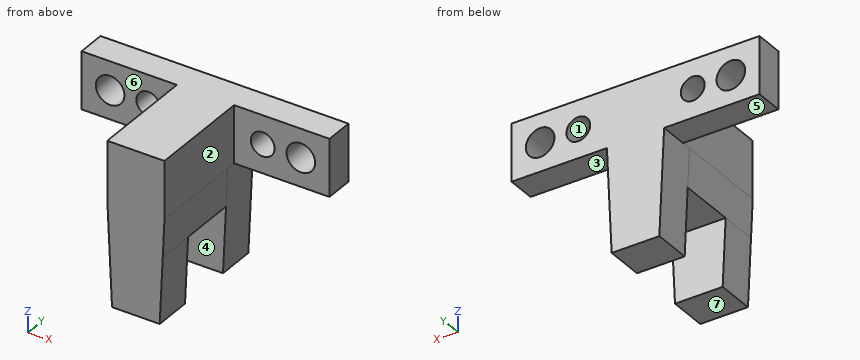
from build123d import *

# Parameters (mm, degrees)
SKETCH_1_W      = 26
SKETCH_1_H      = 6
SKETCH_1_R      = 1.5
SKETCH_1_R_2    = 1.25
EXTRUDE_1_DEPTH = 3
EXTRUDE_2_DEPTH = 4
EXTRUDE_3_DEPTH = 11
EXTRUDE_4_DEPTH = 4


with BuildPart() as part:
    # 草图1 → 凸台-拉伸1 (new body)
    with BuildSketch(Plane(origin=(0, 0, 0), x_dir=(1, 0, 0), z_dir=(0, 1, 0))):
        Rectangle(SKETCH_1_W, SKETCH_1_H)
        with Locations(Location((-10, 0, 0), (0, 0, 270))):
            Circle(SKETCH_1_R, mode=Mode.SUBTRACT)
        with Locations(Location((-6, 0, 0), (0, 0, 270))):
            Circle(SKETCH_1_R_2, mode=Mode.SUBTRACT)
        with Locations(Location((10, 0, 0), (0, 0, 270))):
            Circle(SKETCH_1_R, mode=Mode.SUBTRACT)
        with Locations(Location((6, 0, 0), (0, 0, 270))):
            Circle(SKETCH_1_R_2, mode=Mode.SUBTRACT)
    extrude(amount=EXTRUDE_1_DEPTH)

    # 草图2 → 凸台-拉伸2 (add)
    with BuildSketch(Plane(origin=(0, 3, 0), x_dir=(1, 0, 0), z_dir=(0, 1, 0))):
        Polygon((0, 14), (0, 3), (3, 3), (2.5, 14), align=None)
        Polygon((-3, 3), (0, 3), (0, 14), (-2.5, 14), align=None)
    extrude(amount=-EXTRUDE_2_DEPTH)

    # 草图3 → 凸台-拉伸3 (add)
    with BuildSketch(Plane.XZ):
        Polygon((2.818181818, -7), (3, -3), (0, -3), (0, -7), align=None)
        Polygon((0, -3), (-3, -3), (-2.818181818, -7), (0, -7), align=None)
        Polygon((3, 3), (-3, 3), (-3, -3), (0, -3), (3, -3), align=None)
    extrude(amount=EXTRUDE_3_DEPTH)

    # 草图4 → 凸台-拉伸4 (add)
    with BuildSketch(Plane.XZ.offset(11)):
        Polygon((-2.5, -14), (2.5, -14), (2.818181818, -7), (-2.818181818, -7), align=None)
    extrude(amount=-EXTRUDE_4_DEPTH)


solid = part.part
Read the model definition and answer for the solid it produces. Units are mm, in the model's axes. Face numbers are marked on the shaded views. A direction names the side the tool comes from. Give positions to 0.01 mm unless a question says otherwise; leave off trailing zeros. Write each loop counter-clockwise with the first axis right and the second up, starting at its lowest first coordinate (ties: lowest second). Pieces come first, ordered by that corner, then holes. Notation, with made-up numbers: M 55.25,-21.75 L 95.25,-21.75 A22 cw 95.25,-7.75 Z; hole C -6.75,22.5 d2. An arc over 180 degrees is marked long. One line per item, written item: value. Start each with the question number.
(1) Find section D-D (x = 10). Determine the outline of the cut face in (y, z).
(2) Find the intervals of material crossed by line 1 (X direction, y = 2.3, z = 0); line 2 (Y direction, x = -1.5, z = -9.25); line 3 (Y direction, x = -6.5, z = -2.5), in increasing order.
(3) Find section B-B (z = 0). Determine the outline of the cut face in (x, y).
(4) Find section A-A (x = 6). Determine the outline of the cut face in (y, z), plus the area to 3 significant figures.
(5) A tool of negligible diameter and unlimited length cuts with its end or side. For the marked faces 4, 5, 6 and 7, from which of +Z, -Z, +X, -X, +Y, -Y can it reach the whole face along a straight path? Write none if from no direction.
(6) Find section C-C (y = 1.25). Determine the outline of the cut face in (x, z).
(7) Flat-ended cylindrical pins translate along their axes: pin 1 Ø8 at (y, z) = (0, -11) entering from +X; pin 2 Ø1.5 at (x, y) = (-7, 1.5) entering from -Z; pin 3 Ø3.5 at (x, z) = (10, 0) entering from -Y; pin 4 Ø2 at (x, z) = (6, 0) entering from +Y. Find the tip coordinate at first contact, or state that the pin passes through.
(8) Determine the mould class of the marked faces 1, 2 and 3 for opening direction Z: pulls with the +Z half, pulls with the -Z half, needs draft (parallel to the pull), parting line crosses it, or undercut.
Results below:
1. outline: M 0,-3 L 3,-3 L 3,-1.5 L 0,-1.5 Z; M 0,1.5 L 3,1.5 L 3,3 L 0,3 Z
2. line 1: x = -13 to -11.5, -8.5 to -7.25, -4.75 to 4.75, 7.25 to 8.5, 11.5 to 13
2. line 2: y = -11 to -7, -1 to 3
2. line 3: y = 0 to 3
3. outline: M -13,0 L -11.5,0 L -11.5,3 L -13,3 Z; M -8.5,0 L -7.25,0 L -7.25,3 L -8.5,3 Z; M -4.75,0 L -3,0 L -3,-11 L 3,-11 L 3,0 L 4.75,0 L 4.75,3 L -4.75,3 Z; M 7.25,0 L 8.5,0 L 8.5,3 L 7.25,3 Z; M 11.5,0 L 13,0 L 13,3 L 11.5,3 Z
4. outline: M 0,-3 L 3,-3 L 3,-1.25 L 0,-1.25 Z; M 0,1.25 L 3,1.25 L 3,3 L 0,3 Z
4. area: 10.5 mm^2
5. face 4: -Z, +X, -X
5. face 5: -Z, -X, +Y, -Y
5. face 6: +Z, -Z, -X, -Y
5. face 7: -Z, +X, -X, +Y, -Y
6. outline: M -13,-3 L -3,-3 L -2.5,-14 L 2.5,-14 L 3,-3 L 13,-3 L 13,3 L -13,3 Z; hole C -10,0 d3; hole C -6,0 d2.5; hole C 6,0 d2.5; hole C 10,0 d3
7. pin 1: stops at x = 2.82
7. pin 2: stops at z = -3
7. pin 3: stops at y = 0
7. pin 4: passes through
8. face 1: undercut
8. face 2: needs draft
8. face 3: pulls with the -Z half
